For this review, take the finished solid that the model builds, in its own axes (mm). A direction names the side the tool comes from. Coordinates: 2 decimals unless noted, no trailing zeros. Put each result on its own line as item: value. Start each with the question number.
Item 1: To check wall thickness, follow L1, parallel to X at y = 22.5, z = 9; L2, parallel to X at y = 77, z = 6. State the ranges of each line that lie inside material, in increasing order.
Item 2: The part is to be moulded in two halves that separate along Y. For faces 4 (the flat face through (138, 101.6, 6)), 5 (the flat face through (276, 78.359, 6)), 6 (the flat face through (0, 90, 6)), 7 (the flat face through (4, 23.241, 6)), say which applies: +Y half, -Y half, draft (parallel to the pull), parting line (faces both ways), or undercut.
Item 3: Insertion check: P1, Ø3.5, axis at y = 76, z = 8.5, coming from the +X side. The pin has a flat end and moves straight along its axis. Give the tip position at first contact, or say it passes through.
Item 4: For faces 1 (the flat face through (0, 11, 6)), 2 (the flat face through (4, 27.559, 6)), 3 (the flat face through (276, 23.241, 6)), list the 3-axis set-ups (+Z, -Z, +X, -X, +Y, -Y) from which the entire face can be reached by the end or side of a thin tool; tool diameter is ignored.
```python
from build123d import *

# Parameters (mm, degrees)
SKETCH1_W           = 279.4
SKETCH1_H           = 101.6
BOSS_EXTRUDE1_DEPTH = 12.7
CUT_EXTRUDE1_DEPTH  = 298.570512652


with BuildPart() as part:
    # Sketch1 → Boss-Extrude1 (new body)
    with BuildSketch(Plane.XY):
        with Locations((139.7, 50.8)):
            Rectangle(SKETCH1_W, SKETCH1_H)
    extrude(amount=BOSS_EXTRUDE1_DEPTH)

    # Sketch2 → Cut-Extrude1 (cut, through all)
    with BuildSketch(Plane.XY.offset(12.7)):
        Polygon((279.4, 78.359), (279.4, 74.041), (271.78, 74.041), (271.78, 72.517), (268.478, 72.517), (268.478, 74.041), (264.16, 74.041), (264.16, 78.359), (268.478, 78.359), (268.478, 79.883), (271.78, 79.883), (271.78, 78.359), align=None)
        Polygon((271.78, 23.241), (279.4, 23.241), (279.4, 27.559), (271.78, 27.559), (271.78, 29.083), (268.478, 29.083), (268.478, 27.559), (264.16, 27.559), (264.16, 23.241), (268.478, 23.241), (268.478, 21.717), (271.78, 21.717), align=None)
        Polygon((0, 23.241), (0, 27.559), (7.62, 27.559), (7.62, 29.083), (10.922, 29.083), (10.922, 27.559), (15.24, 27.559), (15.24, 23.241), (10.922, 23.241), (10.922, 21.717), (7.62, 21.717), (7.62, 23.241), align=None)
        Polygon((7.62, 78.359), (0, 78.359), (0, 74.041), (7.62, 74.041), (7.62, 72.517), (10.922, 72.517), (10.922, 74.041), (15.24, 74.041), (15.24, 78.359), (10.922, 78.359), (10.922, 79.883), (7.62, 79.883), align=None)
    extrude(amount=-CUT_EXTRUDE1_DEPTH, mode=Mode.SUBTRACT)


solid = part.part
```
Return value:
1. L1: 0 to 7.62, 10.92 to 268.48, 271.78 to 279.4
1. L2: 15.24 to 264.16
2. face 4: +Y half
2. face 5: undercut
2. face 6: draft
2. face 7: undercut
3. P1: x = 264.16
4. face 1: +Z, -Z, -X, +Y, -Y
4. face 2: +Z, -Z, -X
4. face 3: +Z, -Z, +X
